The listing builds one solid part. Answer for the finished solid, in the listing's coordinates (mm). Face numbers are marked on the shaded views. A direction names the side the tool comes from. Coordinates: 2 decimals unless noted, no trailing zeros. Loops run counter-clockwise (first coordinate to the right, second up) from the corner with the lowest first, then second, coordinate; pieces in that order, holes last. Notation, with made-up numbers: M 42,-3 L 48,-3 A17 ccw 48,11 Z; hole C 9,53.25 d7. An arc over 180 degrees is marked long. Return JSON: item names as keys, results as strings. Group by question number.
1. Section B-B (y = 0) is taken. Write down the section's boundary in (x, z), then the cut area to 3 significant figures.
2. The mould has two halves that part along X. Classify the marked faces 6, 7 and 8: pulls with the +X half, pulls with the -X half, needs draft (parallel to the pull), parting line crosses it, or undercut.
3. Section D-D (x = -7) is taken. Write down the section's boundary in (y, z), then the cut area to 3 significant figures.
4. Section A-A (z = -9.5) is taken. Write down the section's boundary in (x, y), then the cut area to 3 significant figures.
5. Given P1, Ø7.5, axis at y = 0, z = 12.5, coming from the +X side; P2, Ø11, axis at x = 0, y = 0, coming from the -Z side; P3, Ø2, axis at x = 1, z = 5, coming from the +Y side, each flat-ended and moving along its own axis, determine where each tip first touches the part or whether it passes through.
6. Straight lines are drawn through the part: L1, parallel to Y at x = 0, z = 8; L2, parallel to X at y = 0, z = 3. For each, find the intervals that lie inside material, in ascending order. Write a range as from..to.
7. Which of the six approach directions +Z, -Z, +X, -X, +Y, -Y give full straight-line access (tool end or side, diameter ignored) to the marked faces 1, 2, 3, 4 and 5?
```python
from build123d import *

# Parameters (mm, degrees)
SKETCH1_R          = 3.4036
EXTRUDE1_DEPTH     = 20
CUT_EXTRUDE1_DEPTH = 49.989794856


with BuildPart() as part:
    # Sketch1 → Extrude1 (new, symmetric)
    with BuildSketch(Plane.XY):
        with BuildLine():
            Line((-20, 16.952), (-20, 4.7625))
            ThreePointArc((-20, 4.7625), (-19.776815367, 4.223684633), (-19.238, 4.0005))
            Line((-19.238, 4.0005), (-16.2662, 4.0005))
            ThreePointArc((-16.2662, 4.0005), (-15.727384633, 4.223684633), (-15.5042, 4.7625))
            Line((-15.5042, 4.7625), (-15.5042, 10.485558599))
            ThreePointArc((-15.5042, 10.485558599), (-15.033804775, 11.189554802), (-14.203384633, 11.024373966))
            Line((-14.203384633, 11.024373966), (-8.635059555, 5.456048889))
            ThreePointArc((-8.635059555, 5.456048889), (-7.985348265, 4.483687227), (-7.7572, 3.336708444))
            Line((-7.7572, 3.336708444), (-7.7572, -3.336708444))
            ThreePointArc((-7.7572, -3.336708444), (-7.985348265, -4.483687227), (-8.635059555, -5.456048889))
            Line((-8.635059555, -5.456048889), (-14.203384633, -11.024373966))
            ThreePointArc((-14.203384633, -11.024373966), (-15.033804775, -11.189554802), (-15.5042, -10.485558599))
            Line((-15.5042, -10.485558599), (-15.5042, -4.7625))
            ThreePointArc((-15.5042, -4.7625), (-15.727384633, -4.223684633), (-16.2662, -4.0005))
            Line((-16.2662, -4.0005), (-19.238, -4.0005))
            ThreePointArc((-19.238, -4.0005), (-19.776815367, -4.223684633), (-20, -4.7625))
            Line((-20, -4.7625), (-20, -16.952))
            ThreePointArc((-20, -16.952), (-19.107261469, -19.107261469), (-16.952, -20))
            Line((-16.952, -20), (-4.7625, -20))
            ThreePointArc((-4.7625, -20), (-4.223684633, -19.776815367), (-4.0005, -19.238))
            Line((-4.0005, -19.238), (-4.0005, -16.2662))
            ThreePointArc((-4.0005, -16.2662), (-4.223684633, -15.727384633), (-4.7625, -15.5042))
            Line((-4.7625, -15.5042), (-10.485558599, -15.5042))
            ThreePointArc((-10.485558599, -15.5042), (-11.189554802, -15.033804775), (-11.024373966, -14.203384633))
            Line((-11.024373966, -14.203384633), (-5.456048889, -8.635059555))
            ThreePointArc((-5.456048889, -8.635059555), (-4.483687227, -7.985348265), (-3.336708444, -7.7572))
            Line((-3.336708444, -7.7572), (3.336708444, -7.7572))
            ThreePointArc((3.336708444, -7.7572), (4.483687227, -7.985348265), (5.456048889, -8.635059555))
            Line((5.456048889, -8.635059555), (11.024373966, -14.203384633))
            ThreePointArc((11.024373966, -14.203384633), (11.189554802, -15.033804775), (10.485558599, -15.5042))
            Line((10.485558599, -15.5042), (4.7625, -15.5042))
            ThreePointArc((4.7625, -15.5042), (4.223684633, -15.727384633), (4.0005, -16.2662))
            Line((4.0005, -16.2662), (4.0005, -19.238))
            ThreePointArc((4.0005, -19.238), (4.223684633, -19.776815367), (4.7625, -20))
            Line((4.7625, -20), (16.952, -20))
            ThreePointArc((16.952, -20), (19.107261469, -19.107261469), (20, -16.952))
            Line((20, -16.952), (20, -4.7625))
            ThreePointArc((20, -4.7625), (19.776815367, -4.223684633), (19.238, -4.0005))
            Line((19.238, -4.0005), (16.2662, -4.0005))
            ThreePointArc((16.2662, -4.0005), (15.727384633, -4.223684633), (15.5042, -4.7625))
            Line((15.5042, -4.7625), (15.5042, -10.485558599))
            ThreePointArc((15.5042, -10.485558599), (15.033804775, -11.189554802), (14.203384633, -11.024373966))
            Line((14.203384633, -11.024373966), (8.635059555, -5.456048889))
            ThreePointArc((8.635059555, -5.456048889), (7.985348265, -4.483687227), (7.7572, -3.336708444))
            Line((7.7572, -3.336708444), (7.7572, 3.336708444))
            ThreePointArc((7.7572, 3.336708444), (7.985348265, 4.483687227), (8.635059555, 5.456048889))
            Line((8.635059555, 5.456048889), (14.203384633, 11.024373966))
            ThreePointArc((14.203384633, 11.024373966), (15.033804775, 11.189554802), (15.5042, 10.485558599))
            Line((15.5042, 10.485558599), (15.5042, 4.7625))
            ThreePointArc((15.5042, 4.7625), (15.727384633, 4.223684633), (16.2662, 4.0005))
            Line((16.2662, 4.0005), (19.238, 4.0005))
            ThreePointArc((19.238, 4.0005), (19.776815367, 4.223684633), (20, 4.7625))
            Line((20, 4.7625), (20, 16.952))
            ThreePointArc((20, 16.952), (19.107261469, 19.107261469), (16.952, 20))
            Line((16.952, 20), (4.7625, 20))
            ThreePointArc((4.7625, 20), (4.223684633, 19.776815367), (4.0005, 19.238))
            Line((4.0005, 19.238), (4.0005, 16.2662))
            ThreePointArc((4.0005, 16.2662), (4.223684633, 15.727384633), (4.7625, 15.5042))
            Line((4.7625, 15.5042), (10.485558599, 15.5042))
            ThreePointArc((10.485558599, 15.5042), (11.189554802, 15.033804775), (11.024373966, 14.203384633))
            Line((11.024373966, 14.203384633), (5.456048889, 8.635059555))
            ThreePointArc((5.456048889, 8.635059555), (4.483687227, 7.985348265), (3.336708444, 7.7572))
            Line((3.336708444, 7.7572), (-3.336708444, 7.7572))
            ThreePointArc((-3.336708444, 7.7572), (-4.483687227, 7.985348265), (-5.456048889, 8.635059555))
            Line((-5.456048889, 8.635059555), (-11.024373966, 14.203384633))
            ThreePointArc((-11.024373966, 14.203384633), (-11.189554802, 15.033804775), (-10.485558599, 15.5042))
            Line((-10.485558599, 15.5042), (-4.7625, 15.5042))
            ThreePointArc((-4.7625, 15.5042), (-4.223684633, 15.727384633), (-4.0005, 16.2662))
            Line((-4.0005, 16.2662), (-4.0005, 19.238))
            ThreePointArc((-4.0005, 19.238), (-4.223684633, 19.776815367), (-4.7625, 20))
            Line((-4.7625, 20), (-16.952, 20))
            ThreePointArc((-16.952, 20), (-19.107261469, 19.107261469), (-20, 16.952))
        make_face()
        Circle(SKETCH1_R, mode=Mode.SUBTRACT)
    extrude(amount=EXTRUDE1_DEPTH, both=True)

    # Sketch3 → Cut-Extrude1 (cut, through all)
    with BuildSketch(Plane.XZ.offset(20)):
        Polygon((20, 20), (-20, -20), (20, -20), align=None)
    extrude(amount=-CUT_EXTRUDE1_DEPTH, mode=Mode.SUBTRACT)


solid = part.part
```
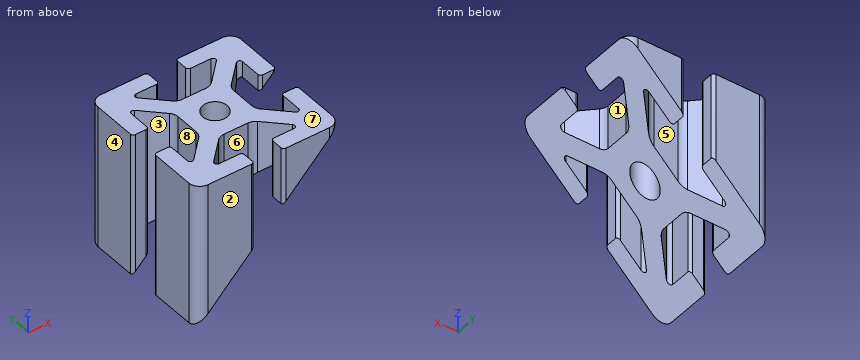
Worked out:
{
 "1": {"outline": "M -7.76,-7.76 L -3.4,-3.4 L -3.4,20 L -7.76,20 Z; M 3.4,3.4 L 7.76,7.76 L 7.76,20 L 3.4,20 Z", "area": "174 mm^2"},
 "2": {"face 6": "undercut", "face 7": "needs draft", "face 8": "pulls with the -X half"},
 "3": {"outline": "M -20,-7 L -15.5,-7 L -15.5,20 L -20,20 Z; M -10.18,-7 L 10.18,-7 L 10.18,20 L -10.18,20 Z; M 15.5,-7 L 20,-7 L 20,20 L 15.5,20 Z", "area": "792 mm^2"},
 "4": {"outline": "M -20,-16.95 A3.05 ccw -16.95,-20 L -9.5,-20 L -9.5,-15.5 L -10.49,-15.5 A0.76 cw -11.02,-14.2 L -9.5,-12.68 L -9.5,-6.32 L -14.2,-11.02 A0.76 cw -15.5,-10.49 L -15.5,-4.76 A0.76 ccw -16.27,-4 L -19.24,-4 A0.76 ccw -20,-4.76 Z; M -20,4.76 A0.76 ccw -19.24,4 L -16.27,4 A0.76 ccw -15.5,4.76 L -15.5,10.49 A0.76 cw -14.2,11.02 L -9.5,6.32 L -9.5,12.68 L -11.02,14.2 A0.76 cw -10.49,15.5 L -9.5,15.5 L -9.5,20 L -16.95,20 A3.05 ccw -20,16.95 Z", "area": "262 mm^2"},
 "5": {"P1": "x = 7.79", "P2": "z = -5.5", "P3": "y = 7.76"},
 "6": {"L1": "-7.76..-3.4, 3.4..7.76", "L2": "-7.76..-3.4"},
 "7": {"face 1": "+Z, -Z, +X", "face 2": "+Z, -Z, +X, -X, -Y", "face 3": "+Z, -Z", "face 4": "+Z, -Z, -X, +Y, -Y", "face 5": "+Z, -Z, +Y"}
}
